```python
from build123d import *

# Parameters (mm, degrees)
F1_DEPTH = 3.175
F2_R     = 5.08
F4_DEPTH = 25.4
F5_R     = 5.08


with BuildPart() as f1:
    # F0 (on Front) → F1 (new body)
    with BuildSketch(Plane.XZ):
        Polygon((-76.2, 0), (0, 0), (-76.2, 76.2), align=None)
    extrude(amount=F1_DEPTH)

    # F2
    f2_edges = [f1.edges().sort_by_distance(p)[0] for p in [
        (-76.2, -1.5875, 76.2),
        (-76.2, -1.5875, 0),
        (0, -1.5875, 0),
    ]]
    fillet(f2_edges, radius=F2_R)

    # F3 (on face) → F4 (cut)
    with BuildSketch(Plane.XZ.offset(3.175)):
        Polygon((-71.12, 38.1), (-71.12, 5.08), (-45.72, 38.1), align=None)
    extrude(amount=-F4_DEPTH, mode=Mode.SUBTRACT)

    # F5
    f5_edges = [f1.edges().sort_by_distance(p)[0] for p in [
        (-71.12, -1.5875, 5.08),
        (-45.72, -1.5875, 38.1),
        (-71.12, -1.5875, 38.1),
    ]]
    fillet(f5_edges, radius=F5_R)


solid = f1.part
```
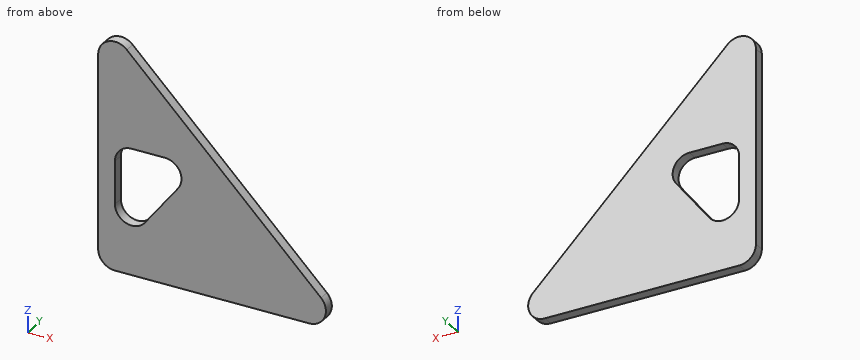
The listing builds one solid part. Answer for the finished solid, in the listing's coordinates (mm). Give positions to 0.01 mm unless a question says otherwise; leave off trailing zeros. Order: outer loops, then holes, each group sorted by start corner. A loop starts at its lowest first (then second) coordinate and runs counter-clockwise, first axis right, second up. Notation, with made-up numbers: (10.5, -38.5) -> (37.5, -38.5) arc R18 ccw to (37.5, -7.5) -> close; hole circle Ø7 at (-23, -4.5). An arc over 180 degrees is marked (long way). Answer as a JSON object with one key per item and string values. Group by question number.
Item 1: Consider L1, parallel to X at y = -1.25, z = 36.5; L2, parallel to Z at x = -63, y = -1.3; L3, parallel to X at y = -2.5, z = 18. Determine where each line is inside the solid, lowest interval first. Write a range as from..to.
Item 2: The part is cut by section D-D on z = 62. Write down the section's boundary in (x, y) (3 decimals).
Item 3: A flat-ended cylindrical pin translates along its axis: pin 1 (1.6 mm diameter, centred on y = -2.5, z = 29.5, fed in from +X). Find the tip coordinate at first contact, or state that the pin passes through.
Item 4: The part is cut by section C-C on x = -64. Write down the section's boundary in (y, z) (3 decimals), and give its area (3 significant figures).
Item 5: The part is cut by section B-B on y = -1.8. Write down the section's boundary in (x, z).
Item 6: The part is cut by section A-A on z = 29. Write down the section's boundary in (x, y) (3 decimals).
Result set:
{
 "1": {"L1": "-76.2..-69.74, -52.34..-36.5", "L2": "0..15.95, 38.1..63", "L3": "-76.2..-70.7, -61.18..-18"},
 "2": {"outline": "(-76.2, -3.175) -> (-62, -3.175) -> (-62, 0) -> (-76.2, 0) -> close"},
 "3": {"pin 1": "x = -28.7"},
 "4": {"outline": "(-3.175, 0) -> (0, 0) -> (0, 15.363) -> (-3.175, 15.363) -> close; (-3.175, 38.1) -> (0, 38.1) -> (0, 64) -> (-3.175, 64) -> close", "area": "131 mm²"},
 "5": {"outline": "(-76.2, 5.08) arc R5.08 ccw to (-71.12, 0) -> (-12.26, 0) arc R5.08 ccw to (-8.67, 8.67) -> (-67.53, 67.53) arc R5.08 ccw to (-76.2, 63.94) -> close; hole (-71.12, 20.02) arc R5.08 ccw to (-62.01, 16.92) -> (-52.01, 29.92) arc R5.08 ccw to (-56.04, 38.1) -> (-66.04, 38.1) arc R5.08 ccw to (-71.12, 33.02) -> close"},
 "6": {"outline": "(-76.2, -3.175) -> (-71.12, -3.175) -> (-71.12, 0) -> (-76.2, 0) -> close; (-52.72, -3.175) -> (-29, -3.175) -> (-29, 0) -> (-52.72, 0) -> close"}
}
